Model file for the job. Use its own axes, mm. Face numbers are marked on the shaded views. A direction names the side the tool comes from. Round coordinates to 2 decimals unless told otherwise and drop trailing zeros. Loops run counter-clockwise (first coordinate to the right, second up) from the corner with the lowest first, then second, coordinate; pieces in that order, holes last. Notation, with made-up numbers: (-3, -39.5) - (51, -39.5) arc R35 ccw to (51, -1.5) - close; hole circle Ø8 at (54, 39). An arc over 180 degrees is marked (long way). Answer as a JSON object with one key per item and string values.
from build123d import *

# Parameters (mm, degrees)
SKETCH_1_R          = 30
EXTRUDE_1_DEPTH     = 30
SKETCH_2_R          = 3.5
EXTRUDE_2_DEPTH     = 7
SKETCH_3_R          = 24
CUT_EXTRUDE_1_DEPTH = 26
SKETCH_4_R          = 3.5
CUT_EXTRUDE_2_DEPTH = 60.063525123
SKETCH_5_R          = 8.5
SKETCH_5_R_2        = 7.5
CUT_EXTRUDE_3_DEPTH = 2.5
CHAMFER_1_SIZE      = 0.5
SKETCH_10_W         = 12
SKETCH_10_H         = 8
CUT_EXTRUDE_4_DEPTH = 49
SKETCH_11_R         = 25
SKETCH_11_R_2       = 17.5
EXTRUDE_3_DEPTH     = 2.5
FILLET_1_R          = 1


with BuildPart() as part:
    # 草图1 → 凸台-拉伸1 (new body)
    with BuildSketch(Plane(origin=(0, 0, 0), x_dir=(1, 0, 0), z_dir=(0, 1, 0))):
        with Locations(Location((0, 0, 0), (0, 0, 270))):
            Circle(SKETCH_1_R)
    extrude(amount=EXTRUDE_1_DEPTH)

    # 草图2 → 凸台-拉伸2 (add)
    with BuildSketch(Plane.XZ):
        with BuildLine():
            Line((-27.5, -37.5), (27.5, -37.5))
            ThreePointArc((27.5, -37.5), (34.571067812, -34.571067812), (37.5, -27.5))
            Line((37.5, -27.5), (37.5, 27.5))
            ThreePointArc((37.5, 27.5), (34.571067812, 34.571067812), (27.5, 37.5))
            Line((27.5, 37.5), (-27.5, 37.5))
            ThreePointArc((-27.5, 37.5), (-34.571067812, 34.571067812), (-37.5, 27.5))
            Line((-37.5, 27.5), (-37.5, -27.5))
            ThreePointArc((-37.5, -27.5), (-34.571067812, -34.571067812), (-27.5, -37.5))
        make_face()
        with Locations(Location((-24.999998784, 24.999998784, 0), (0, 0, 270))):
            Circle(SKETCH_2_R, mode=Mode.SUBTRACT)
        with Locations(Location((-25.000001216, -25.000001216, 0), (0, 0, 270))):
            Circle(SKETCH_2_R, mode=Mode.SUBTRACT)
        with Locations(Location((25.000001216, 25.000001216, 0), (0, 0, 270))):
            Circle(SKETCH_2_R, mode=Mode.SUBTRACT)
        with Locations(Location((24.999998784, -24.999998784, 0), (0, 0, 270))):
            Circle(SKETCH_2_R, mode=Mode.SUBTRACT)
    extrude(amount=-EXTRUDE_2_DEPTH)

    # 草图3 → 切除-拉伸1 (cut)
    with BuildSketch(Plane.XZ):
        with Locations(Location((0, 0, 0), (0, 0, 270))):
            Circle(SKETCH_3_R)
    extrude(amount=-CUT_EXTRUDE_1_DEPTH, mode=Mode.SUBTRACT)

    # 草图4 → 切除-拉伸2 (cut, through all)
    with BuildSketch(Plane.XZ.offset(-26)):
        with Locations(Location((0, 0, 0), (0, 0, 270))):
            Circle(SKETCH_4_R)
    extrude(amount=-CUT_EXTRUDE_2_DEPTH, mode=Mode.SUBTRACT)

    # 草图5 → 切除-拉伸3 (cut)
    with BuildSketch(Plane.XZ.offset(-26)):
        with Locations(Location((0, 0, 0), (0, 0, 270))):
            Circle(SKETCH_5_R)
        with Locations(Location((0, 0, 0), (0, 0, 270))):
            Circle(SKETCH_5_R_2, mode=Mode.SUBTRACT)
    extrude(amount=-CUT_EXTRUDE_3_DEPTH, mode=Mode.SUBTRACT)

    # 倒角1
    chamfer_1_edges = [part.edges().sort_by_distance(p)[0] for p in [
        (0, 26, 3.5),
    ]]
    chamfer(chamfer_1_edges, length=CHAMFER_1_SIZE)

    # 草图10 → 切除-拉伸4 (cut)
    with BuildSketch(Plane.XY):
        with Locations((0, 19)):
            Rectangle(SKETCH_10_W, SKETCH_10_H)
    extrude(amount=-CUT_EXTRUDE_4_DEPTH, mode=Mode.SUBTRACT)

    # 草图11 → 凸台-拉伸3 (add)
    with BuildSketch(Plane(origin=(0, 30, 0), x_dir=(1, 0, 0), z_dir=(0, 1, 0))):
        with Locations(Location((0, 0, 0), (0, 0, 270))):
            Circle(SKETCH_11_R)
        with Locations(Location((0, 0, 0), (0, 0, 270))):
            Circle(SKETCH_11_R_2, mode=Mode.SUBTRACT)
    extrude(amount=EXTRUDE_3_DEPTH)

    # 圆角1
    fillet_1_edges = [part.edges().sort_by_distance(p)[0] for p in [
        (0, 30, -30),
        (0, 32.5, -25),
        (0, 32.5, -17.5),
    ]]
    fillet(fillet_1_edges, radius=FILLET_1_R)


solid = part.part
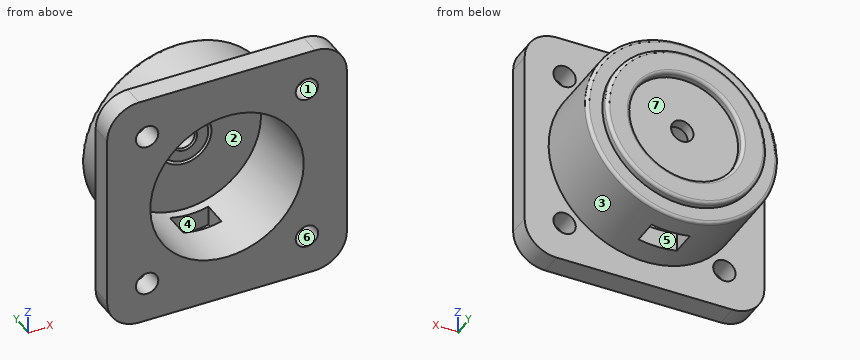
1) Slice it at A-A on y = 3. List the corners of the cut face in (x, z).
Values follow:
{"outline": "(-37.5, -27.5) arc R10 ccw to (-27.5, -37.5) - (27.5, -37.5) arc R10 ccw to (37.5, -27.5) - (37.5, 27.5) arc R10 ccw to (27.5, 37.5) - (-27.5, 37.5) arc R10 ccw to (-37.5, 27.5) - close; hole circle Ø7 at (-25, -25); hole circle Ø7 at (-25, 25); hole circle Ø48 at (0, 0); hole circle Ø7 at (25, -25); hole circle Ø7 at (25, 25)"}
2) Two-plate mould, pull along Y, no slides. Class the marked faces 5, 6 and 7: pulls with the +Y half, pulls with the -Y half, needs draft (parallel to the pull), parting line crosses it, or undercut.
Values follow:
{"face 5": "undercut", "face 6": "needs draft", "face 7": "pulls with the +Y half"}
3) Slice it at B-B on x = 0. Count the separate pieces of the cut face and the enclosed holes in it, then the cut area to 3 significant figures.
Values follow:
{"separate pieces": "3", "enclosed holes": "0", "area": "612 mm²"}
4) Slice it at D-D on z = -31. List the corners of the cut face in (x, y).
Values follow:
{"outline": "(-36.87, 0) - (36.87, 0) - (36.87, 7) - (-36.87, 7) - close"}
5) Slice it at C-C on y = 11. List the corners of the cut face in (x, z), then the cut area to 3 significant figures.
Values follow:
{"outline": "circle Ø60 at (0, 0); hole circle Ø48 at (0, 0)", "area": "1,020 mm²"}
6) Probe probe 1 along X at (y, z) = (31, 0); probe 2 along Y at (x, z) = (-4.5, 30); probe 3 along Y at (x, z) = (-18.5, -10). List the from-to ranges inside material, lowest first.
Values follow:
{"probe 1": "-25 to -17.5, 17.5 to 25", "probe 2": "0 to 7", "probe 3": "26 to 32.5"}
7) Drop flat-ended pins along their axis: P1, Ø3, axis at y = 23.5, z = 1, coming from the +X side; P2, Ø7, axis at y = 17.5, z = -26, coming from the -X side; P3, Ø13.5, axis at x = 2, z = -3, coming from the -Y side. Give the stop position or say it passes through.
Values follow:
{"P1": "x = 30", "P2": "x = -19.84", "P3": "y = 26"}
8) Tool access for the marked faces 1, 2, 3 and 4: list every direction of +Z, -Z, +X, -X, +Y, -Y with a clear straight run to the whole face (end or side of a thin tool).
Values follow:
{"face 1": "+Y, -Y", "face 2": "-Y", "face 3": "+Y", "face 4": "-Z"}
